```python
from build123d import *

# Parameters (mm, degrees)
F1_DEPTH = 25
F3_DEPTH = 3
F4_R     = 1
F5_DEPTH = 3


with BuildPart() as f1:
    # F0 (on Top) → F1 (new body)
    with BuildSketch(Plane.XY):
        with BuildLine():
            Line((0, 20), (0, 15))
            Line((0, 15), (20, 15))
            ThreePointArc((20, 15), (38.2805059355, 17.2682292257), (55, 25))
            Line((55, 25), (70, 35))
            Line((70, 35), (67.2264990189, 39.1602514717))
            Line((67.2264990189, 39.1602514717), (52.2264990189, 29.1602514717))
            ThreePointArc((52.2264990189, 29.1602514717), (36.8313987252, 22.0536192236), (20, 20))
            Line((20, 20), (0, 20))
        make_face()
    extrude(amount=F1_DEPTH)



with BuildPart() as f1b:
    # F0 (on Top) → F1, piece 2 (new body)
    with BuildSketch(Plane.XY):
        with BuildLine():
            Line((20, -15), (0, -15))
            Line((0, -15), (0, -20))
            Line((0, -20), (20, -20))
            ThreePointArc((20, -20), (36.8307254493, -22.4287692466), (52.2881087807, -29.516895921))
            Line((52.2881087807, -29.516895921), (67.2881087807, -39.2006720908))
            Line((67.2881087807, -39.2006720908), (70, -35))
            Line((70, -35), (55, -25.3162238302))
            ThreePointArc((55, -25.3162238302), (38.2443448369, -17.6327625507), (20, -15))
        make_face()
    extrude(amount=F1_DEPTH)


with BuildPart() as f1_1:
    add(f1.part)

    add(f1b.part)  # F3 merges F1b
    # F2 (on Top) → F3 (join)
    with BuildSketch(Plane.XY):
        Polygon((31.2723219395, 17.9464295506), (0, 17.5446420908), (0, -17.1428583562), (26.3169649988, -17.1428583562), (39.7098250687, -20.0892854482), (53.7723265588, -27.187500149), (69.9766278267, -34.9970981479), (69.9766278267, 34.9736848865), (58.1919662654, 30.1339291036), (44.7991117835, 22.7678567171), align=None)
    extrude(amount=F3_DEPTH)

    # F4 (on face) → F5 (cut)
    with BuildSketch(Plane.XY.offset(3)):
        with Locations((15.3143024072, 0)):
            Circle(F4_R)
        with Locations((53.9886541665, 14.5440837368)):
            Circle(F4_R)
        with Locations((53.9886541665, -14.5440837368)):
            Circle(F4_R)
    extrude(amount=-F5_DEPTH, mode=Mode.SUBTRACT)


solid = f1_1.part
```
Input: part model. Units: mm. Frame: model coordinates. A direction names the side the tool comes from. Give positions to 0.01 mm unless a question says otherwise; leave off trailing zeros. Order: outer loops, then holes, each group sorted by start corner. A loop starts at its lowest first (then second) coordinate and runs counter-clockwise, first axis right, second up. Notation, with made-up numbers: M -13.5,-20 L -3.5,-20 A19 cw -3.5,10 Z; hole C 73,31.25 d6. An arc over 180 degrees is marked long. One line per question, with ' | ' between items. Start each with the question number.
1. Pull-direction query (X, two-part tool) for faces 5 (the face through (10, -20, 12)), 6 (the face through (69.977, 0, 1)), 7 (the face through (52.99, 14.59, 1.52)), 8 (the face through (59.7, -34.3, 12.3)); classes: released by +X, released by -X, zero draft, split by the parting line, or undercut.
2. Access query for faces 1 (the face through (62.395, 29.93, 15.103)), 2 (the face through (10, -15, 14)), 3 (the face through (68.625, -37.13, 12.325)), 4 (the face through (10, 20, 12)). Directions: +Z, -Z, +X, -X, +Y, -Y. A direction counts if a zero-diameter tool reaches every point of the face in a straight line with its end or side. Return the directions, or none.
3. Section query A-A (y = 0). Return the cut outline in (x, z).
4. First-contact query: pin 1 Ø10 at (x, z) = (13, 13.5) entering from +Y; pin 2 Ø4 at (x, z) = (26.5, 19) entering from -Y; pin 3 Ø3.5 at (y, z) = (9, 1.5) entering from +X. Flat tips, straight axial feed; report the tip coordinate or a pass-through.
5. Section query C-C (x = 62.5). Return the cut outline in (y, z).
6. Section query B-B (z = 13.5). Return the cut outline in (x, y) (1 decimal).
7. Section query D-D (y = -8.5). Return the cut outline in (x, z), and give its area (3 significant figures).
8. Material intervals for probe 1 along Y at (x, z) = (20, 3.5); probe 2 along Z at (x, y) = (44, -15); probe 3 along Y at (x, z) = (60, 6.75), sorted ascending. Write a range as [from, to].
Here are the results:
1) face 5: zero draft | face 6: released by +X | face 7: undercut | face 8: released by -X
2) face 1: +Z, +X | face 2: +Z, +X, -X | face 3: +Z, -Z, +X, -Y | face 4: +Z, -Z, -X, +Y
3) outline: M 0,0 L 14.31,0 L 14.31,3 L 0,3 Z; M 16.31,0 L 69.98,0 L 69.98,3 L 16.31,3 Z
4) pin 1: y = 20 | pin 2: y = -20.61 | pin 3: x = 69.98
5) outline: M -36.11,0 L 36.01,0 L 36.01,25 L 30,25 L 30,3 L -30.16,3 L -30.16,25 L -36.11,25 Z
6) outline: M 0,-20 L 20,-20 A59.5 cw 52.3,-29.5 L 67.3,-39.2 L 70,-35 L 55,-25.3 A64.5 ccw 20,-15 L 0,-15 Z; M 0,15 L 20,15 A59.7 ccw 55,25 L 70,35 L 67.2,39.2 L 52.2,29.2 A54.7 cw 20,20 L 0,20 Z
7) outline: M 0,0 L 69.98,0 L 69.98,3 L 0,3 Z | area: 210 mm²
8) probe 1: [-20, -15], [15, 20] | probe 2: [0, 3] | probe 3: [-34.5, -28.54], [28.33, 34.34]
